Can you work these out from the model? Positions are in its coordinate system, mm. Face numbers are marked on the shaded views. A direction names the side the tool comes from. Give positions to 0.01 mm unless a question says otherwise; leave off trailing zeros. Order: outer loops, then holes, each group sorted by start corner. A loop starts at its lowest first (then second) coordinate and runs counter-clockwise, first axis right, second up. Notation, with made-up numbers: M 73.5,-36 L 132.5,-36 A23 ccw 132.5,-1 Z; hole C 28,-0.75 d5. An arc over 180 degrees is marked long. One line per question, with ' | ' between items. Start each with the question number.
1) If we section it at B-B, the plane x = 42: Please give me the cut outline in (y, z).
2) If we section it at A-A, the plane y = 0: Please give me the cut outline in (x, z).
3) Please list where these lines run through material, in increasing order: line 1 along Y through (x, z) = (8, 0); line 2 along X through (y, z) = (-1, 2.55); line 3 along X through (y, z) = (1.5, -1). Write a range as [from, to].
4) I'm going to push flat-ended pins straight in: pin 1 Ø3 at (x, z) = (20, 2) entering from -Y; pin 2 Ø1.5 at (y, z) = (0, 0) entering from -X; pin 3 Ø1 at (x, z) = (54, -1.5) entering from -Y. Where does each tip first touch, or does it pass through?
5) For the marked faces 1 and 2, which set-ups out of +Z, -Z, +X, -X, +Y, -Y let a thin tool reach every point of the face, with its end or its side?
```python
from build123d import *

# Parameters (mm, degrees)
BOSS_EXTRUDE1_DEPTH = 60
SKETCH2_R           = 1.5
BOSS_EXTRUDE2_DEPTH = 8
SKETCH3_R           = 1.5
CUT_EXTRUDE1_DEPTH  = 10
CHAMFER1_SIZE       = 0.3


with BuildPart() as part:
    # Sketch1 → Boss-Extrude1 (new body)
    with BuildSketch(Plane(origin=(0, 0, 0), x_dir=(0, 0, -1), z_dir=(1, 0, 0))):
        Polygon((0, 3.175426481), (-2.75, 1.58771324), (-2.75, -1.58771324), (0, -3.175426481), (2.75, -1.58771324), (2.75, 1.58771324), align=None)
    extrude(amount=BOSS_EXTRUDE1_DEPTH)

    # Sketch2 → Boss-Extrude2 (add)
    with BuildSketch(Plane(origin=(60, 0, 0), x_dir=(0, 0, -1), z_dir=(1, 0, 0))):
        Circle(SKETCH2_R)
    extrude(amount=BOSS_EXTRUDE2_DEPTH)

    # Sketch3 → Cut-Extrude1 (cut)
    with BuildSketch(Plane.ZY):
        Circle(SKETCH3_R)
    extrude(amount=-CUT_EXTRUDE1_DEPTH, mode=Mode.SUBTRACT)

    # Sketch4 → Cut-Revolve1 (revolve, cut)
    with BuildSketch(Plane(origin=(0, 0, 0), x_dir=(1, 0, 0), z_dir=(0, 1, 0))):
        Polygon((0, 10.219809024), (4.392081913, 10.219809024), (0, 2.6125), align=None)
        Polygon((60, 2.6125), (60, 10.219809024), (55.607918087, 10.219809024), align=None)
    revolve(axis=Axis((0, 0, 0), (-1, 0, 0)), mode=Mode.SUBTRACT)

    # Chamfer1
    chamfer1_edges = [part.edges().sort_by_distance(p)[0] for p in [
        (68, 0, 1.5),
    ]]
    chamfer(chamfer1_edges, length=CHAMFER1_SIZE)


solid = part.part
```
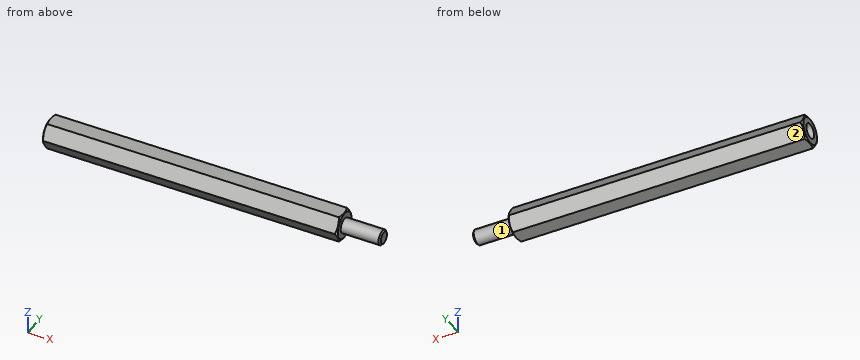
Results found:
1) outline: M -3.18,0 L -1.59,-2.75 L 1.59,-2.75 L 3.18,0 L 1.59,2.75 L -1.59,2.75 Z
2) outline: M 0,-2.61 L 0.08,-2.75 L 59.92,-2.75 L 60,-2.61 L 60,-1.5 L 67.7,-1.5 L 68,-1.2 L 68,1.2 L 67.7,1.5 L 60,1.5 L 60,2.61 L 59.92,2.75 L 0.08,2.75 L 0,2.61 L 0,1.5 L 10,1.5 L 10,-1.5 L 0,-1.5 Z
3) line 1: y = [-3.18, -1.5], [1.5, 3.18] | line 2: x = [0.07, 59.93] | line 3: x = [0, 60]
4) pin 1: stops at y = -2.89 | pin 2: stops at x = 10 | pin 3: stops at y = -2.6
5) face 1: +X | face 2: -Z, +X, -X, +Y
